Part model, mm, in its own coordinate system. A direction names the side the tool comes from. Round coordinates to 2 decimals unless told otherwise and drop trailing zeros. Write each loop counter-clockwise with the first axis right and the second up, starting at its lowest first coordinate (ties: lowest second). Pieces come first, ordered by that corner, then holes. Notation, with made-up numbers: M 14,-29.5 L 56,-29.5 A33 cw 56,-0.5 Z; hole C 74,3.5 d6. An arc over 180 degrees is marked long. Use a Markdown table: item, result. Add a question column.
1) Which spindle directions (+Z, -Z, +X, -X, +Y, -Y) get a long thin tool onto all of the face, cutting with end or side? Do faces 1 (the face through (0, 16, 12.7)), 2 (the face through (190.589, 9.965, 196.939)), 3 (the face through (0.09, -10.07, 6.26)). Say none if no direction does.
2) Two-plate mould, pull along Y, no slides. Class faces 4 (the face through (190.41, -10.07, 196.94)), 5 (the face through (6.35, 0, 94)), 6 (the face through (48.7, -12.7, 148.1)), 7 (the face through (0.09, 5.8, 158.05)): released by +Y, released by -Y, zero draft, split by the parting line, or undercut.
3) Slice it at A-A on z = 142.5. Write the cut outline in (x, y).
4) Slice it at D-D on x = 154. Write the cut outline in (y, z), plus the area to 3 significant figures.
5) Slice it at C-C on y = 0. Write the cut outline in (x, z).
6) Wall check: probe 1 along Z at (x, y) = (-1, 6); probe 2 along X at (y, z) = (6, 197); probe 3 along Z at (x, y) = (56, 1.5). Give the ranges that are in metal, low to high.
7) Drop flat-ended pins along their axis: P1, Ø4, axis at x = 25.5, y = -14, coming from the -Z side; P2, Ø15, axis at x = 110.5, y = -3.5, coming from the -Z side; P3, Ø1, axis at y = -3, z = 146, coming from the +X side; P4, Ø6.5, axis at x = -3, y = -15.5, coming from the -Z side. Give the stop position or say it passes through.
8) Slice it at B-B on x = 55. Write the cut outline in (y, z).
```python
from build123d import *

# Parameters (mm, degrees)
SKETCH1_W           = 12.7
SKETCH1_H           = 50.8
BOSS_EXTRUDE1_DEPTH = 203.2
SKETCH2_W           = 12.7
SKETCH2_H           = 50.8
BOSS_EXTRUDE2_DEPTH = 190.5
BOSS_EXTRUDE5_DEPTH = 12.7
CUT_EXTRUDE2_DEPTH  = 285.051619429
CUT_EXTRUDE3_DEPTH  = 280.688487428
SKETCH9_R           = 2.54
CUT_EXTRUDE4_DEPTH  = 276.109673585
SKETCH10_R          = 2.54
CUT_EXTRUDE5_DEPTH  = 280.688487428


with BuildPart() as part:
    # Sketch1 → Boss-Extrude1 (new body)
    with BuildSketch(Plane.XY):
        Rectangle(SKETCH1_W, SKETCH1_H)
    extrude(amount=BOSS_EXTRUDE1_DEPTH)

    # Sketch2 → Boss-Extrude2 (add)
    with BuildSketch(Plane(origin=(6.35, 0, 0), x_dir=(0, 0, -1), z_dir=(1, 0, 0))):
        with Locations((-196.85, 0)):
            Rectangle(SKETCH2_W, SKETCH2_H)
    extrude(amount=BOSS_EXTRUDE2_DEPTH)

    # Sketch6 → Boss-Extrude5 (add)
    with BuildSketch(Plane.XZ.offset(25.4)):
        Polygon((6.35, 114.3), (6.35, 105.319743879), (91.530256121, 190.5), (82.55, 190.5), align=None)
    extrude(amount=-BOSS_EXTRUDE5_DEPTH)

    # Sketch7 → Cut-Extrude2 (cut, through all)
    with BuildSketch(Plane.XY.offset(203.2)):
        Polygon((196.85, 3.666174209), (196.85, 6.35), (184.15, 13.682348419), (184.15, 0), (196.85, 0), align=None)
        Polygon((196.85, 0), (184.15, 0), (184.15, -3.666174209), (184.15, -13.682348419), (196.85, -6.35), align=None)
    extrude(amount=-CUT_EXTRUDE2_DEPTH, mode=Mode.SUBTRACT)

    # Sketch8 → Cut-Extrude3 (cut, through all)
    with BuildSketch(Plane(origin=(6.35, 0, 0), x_dir=(0, 0, -1), z_dir=(1, 0, 0))):
        Polygon((-12.7, 6.35), (0, 13.682348419), (0, 25.4), (-12.7, 25.4), align=None)
        Polygon((0, -25.4), (0, -13.682348419), (-12.7, -6.35), (-12.7, -25.4), align=None)
    extrude(amount=-CUT_EXTRUDE3_DEPTH, mode=Mode.SUBTRACT)

    # Sketch9 → Cut-Extrude4 (cut, through all)
    with BuildSketch(Plane(origin=(0, 0, 190.5), x_dir=(-1, 0, 0), z_dir=(0, 0, -1))):
        with Locations((-36.322, 6.35)):
            Circle(SKETCH9_R)
    extrude(amount=-CUT_EXTRUDE4_DEPTH, mode=Mode.SUBTRACT)

    # Sketch10 → Cut-Extrude5 (cut, through all)
    with BuildSketch(Plane(origin=(6.35, 0, 0), x_dir=(0, 0, -1), z_dir=(1, 0, 0))):
        with Locations(Location((-160.528, 6.35, 0), (0, 0, 90))):
            Circle(SKETCH10_R)
    extrude(amount=-CUT_EXTRUDE5_DEPTH, mode=Mode.SUBTRACT)


solid = part.part
```
Entries:
| question | item | result |
|---|---|---|
| 1 | face 1 | +X, -X, +Y |
| 1 | face 2 | +Z, -Z |
| 1 | face 3 | +X, -X, -Y |
| 2 | face 4 | undercut |
| 2 | face 5 | zero draft |
| 2 | face 6 | released by +Y |
| 2 | face 7 | undercut |
| 3 | outline | M -6.35,-25.4 L 6.35,-25.4 L 6.35,25.4 L -6.35,25.4 Z; M 34.55,-25.4 L 43.53,-25.4 L 43.53,-12.7 L 34.55,-12.7 Z |
| 4 | outline | M -25.4,190.5 L 25.4,190.5 L 25.4,203.2 L -25.4,203.2 Z |
| 4 | area | 645 mm^2 |
| 5 | outline | M -6.35,0 L 6.35,0 L 6.35,190.5 L 184.15,190.5 L 184.15,203.2 L -6.35,203.2 Z |
| 6 | probe 1 | z = 0 to 158.01, 163.04 to 203.2 |
| 6 | probe 2 | x = -6.35 to 33.81, 38.84 to 184.15 |
| 6 | probe 3 | z = 190.5 to 203.2 |
| 7 | P1 | stops at z = 122.47 |
| 7 | P2 | stops at z = 190.5 |
| 7 | P3 | stops at x = 6.35 |
| 7 | P4 | stops at z = 0 |
| 8 | outline | M -25.4,153.97 L -12.7,153.97 L -12.7,162.95 L -25.4,162.95 Z; M -25.4,190.5 L 25.4,190.5 L 25.4,203.2 L -25.4,203.2 Z |
